Could you check a few things on this model? Use its own coordinates, in mm. Face numbers are marked on the shaded views. A direction names the side the tool comes from. Give positions to 0.01 mm unless a question says otherwise; leave off trailing zeros. Order: outer loops, then holes, each group sorted by start corner. A loop starts at its lowest first (then second) coordinate and runs counter-clockwise, first axis right, second up. Notation, with made-up numbers: (42, 66) -> (70, 66) arc R11 cw to (70, 76) -> close; hole circle Ø4 at (58.25, 11). An arc over 180 degrees is marked (long way). One line per item, written item: value.
```python
from build123d import *

# Parameters (mm, degrees)
EXTRUDE_1_DEPTH = 5
FILLET_1_R      = 0.5


with BuildPart() as part:
    # 草图1 → 凸台-拉伸1 (new body)
    with BuildSketch(Plane(origin=(0, 0, 0), x_dir=(1, 0, 0), z_dir=(0, 1, 0))):
        with BuildLine():
            ThreePointArc((-8.316516862, 5.552976435), (-7.071067812, 7.071067812), (-5.552976435, 8.316516862))
            Line((-5.552976435, 8.316516862), (-12.76036541, 15.523905838))
            Line((-12.76036541, 15.523905838), (-15.523905838, 12.76036541))
            Line((-15.523905838, 12.76036541), (-8.316516862, 5.552976435))
        make_face()
        with BuildLine():
            Line((-20, -1.954118176), (-9.807212762, -1.954118176))
            ThreePointArc((-9.807212762, -1.954118176), (-10, 0), (-9.807212762, 1.954118176))
            Line((-9.807212762, 1.954118176), (-20, 1.954118176))
            Line((-20, 1.954118176), (-20, -1.954118176))
        make_face()
        with BuildLine():
            Line((-12.76036541, -15.523905838), (-5.552976435, -8.316516862))
            ThreePointArc((-5.552976435, -8.316516862), (-7.071067812, -7.071067812), (-8.316516862, -5.552976435))
            Line((-8.316516862, -5.552976435), (-15.523905838, -12.76036541))
            Line((-15.523905838, -12.76036541), (-12.76036541, -15.523905838))
        make_face()
        with BuildLine():
            ThreePointArc((-1.954118176, -9.807212762), (-0.981802522, -9.951686481), (0, -10))
            Line((0, -10), (0, -2.5))
            ThreePointArc((0, -2.5), (-2.5, 0), (0, 2.5))
            Line((0, 2.5), (0, 10))
            ThreePointArc((0, 10), (-0.981802522, 9.951686481), (-1.954118176, 9.807212762))
            ThreePointArc((-1.954118176, 9.807212762), (-3.826834324, 9.238795325), (-5.552976435, 8.316516862))
            ThreePointArc((-5.552976435, 8.316516862), (-7.071067812, 7.071067812), (-8.316516862, 5.552976435))
            ThreePointArc((-8.316516862, 5.552976435), (-9.238795325, 3.826834324), (-9.807212762, 1.954118176))
            ThreePointArc((-9.807212762, 1.954118176), (-10, 0), (-9.807212762, -1.954118176))
            ThreePointArc((-9.807212762, -1.954118176), (-9.238795325, -3.826834324), (-8.316516862, -5.552976435))
            ThreePointArc((-8.316516862, -5.552976435), (-7.071067812, -7.071067812), (-5.552976435, -8.316516862))
            ThreePointArc((-5.552976435, -8.316516862), (-3.826834324, -9.238795325), (-1.954118176, -9.807212762))
        make_face()
        with BuildLine():
            Line((0, -2.5), (0, -10))
            ThreePointArc((0, -10), (0.981802522, -9.951686481), (1.954118176, -9.807212762))
            ThreePointArc((1.954118176, -9.807212762), (3.826834324, -9.238795325), (5.552976435, -8.316516862))
            ThreePointArc((5.552976435, -8.316516862), (7.071067812, -7.071067812), (8.316516862, -5.552976435))
            ThreePointArc((8.316516862, -5.552976435), (9.238795325, -3.826834324), (9.807212762, -1.954118176))
            ThreePointArc((9.807212762, -1.954118176), (9.951686481, -0.981802522), (10, 0))
            ThreePointArc((10, 0), (9.951686481, 0.981802522), (9.807212762, 1.954118176))
            ThreePointArc((9.807212762, 1.954118176), (9.238795325, 3.826834324), (8.316516862, 5.552976435))
            ThreePointArc((8.316516862, 5.552976435), (7.071067812, 7.071067812), (5.552976435, 8.316516862))
            ThreePointArc((5.552976435, 8.316516862), (3.826834324, 9.238795325), (1.954118176, 9.807212762))
            ThreePointArc((1.954118176, 9.807212762), (0.981802522, 9.951686481), (0, 10))
            Line((0, 10), (0, 2.5))
            ThreePointArc((0, 2.5), (1.767766953, 1.767766953), (2.5, 0))
            ThreePointArc((2.5, 0), (1.767766953, -1.767766953), (0, -2.5))
        make_face()
        with BuildLine():
            Line((0, 20), (0, 10))
            ThreePointArc((0, 10), (0.981802522, 9.951686481), (1.954118176, 9.807212762))
            Line((1.954118176, 9.807212762), (1.954118176, 20))
            Line((1.954118176, 20), (0, 20))
        make_face()
        with BuildLine():
            ThreePointArc((-1.954118176, 9.807212762), (-0.981802522, 9.951686481), (0, 10))
            Line((0, 10), (0, 20))
            Line((0, 20), (-1.954118176, 20))
            Line((-1.954118176, 20), (-1.954118176, 9.807212762))
        make_face()
        with BuildLine():
            Line((12.76036541, 15.523905838), (5.552976435, 8.316516862))
            ThreePointArc((5.552976435, 8.316516862), (7.071067812, 7.071067812), (8.316516862, 5.552976435))
            Line((8.316516862, 5.552976435), (15.523905838, 12.76036541))
            Line((15.523905838, 12.76036541), (12.76036541, 15.523905838))
        make_face()
        with BuildLine():
            ThreePointArc((10, 0), (9.951686481, -0.981802522), (9.807212762, -1.954118176))
            Line((9.807212762, -1.954118176), (20, -1.954118176))
            Line((20, -1.954118176), (20, 1.954118176))
            Line((20, 1.954118176), (9.807212762, 1.954118176))
            ThreePointArc((9.807212762, 1.954118176), (9.951686481, 0.981802522), (10, 0))
        make_face()
        with BuildLine():
            ThreePointArc((8.316516862, -5.552976435), (7.071067812, -7.071067812), (5.552976435, -8.316516862))
            Line((5.552976435, -8.316516862), (12.76036541, -15.523905838))
            Line((12.76036541, -15.523905838), (15.523905838, -12.76036541))
            Line((15.523905838, -12.76036541), (8.316516862, -5.552976435))
        make_face()
        with BuildLine():
            Line((-1.954118176, -20), (0, -20))
            Line((0, -20), (0, -10))
            ThreePointArc((0, -10), (-0.981802522, -9.951686481), (-1.954118176, -9.807212762))
            Line((-1.954118176, -9.807212762), (-1.954118176, -20))
        make_face()
        with BuildLine():
            Line((0, -10), (0, -20))
            Line((0, -20), (1.954118176, -20))
            Line((1.954118176, -20), (1.954118176, -9.807212762))
            ThreePointArc((1.954118176, -9.807212762), (0.981802522, -9.951686481), (0, -10))
        make_face()
    extrude(amount=EXTRUDE_1_DEPTH)

    # 圆角1
    fillet_1_edges = [part.edges().sort_by_distance(p)[0] for p in [
        (9.156670922, 5, 11.92021135),
        (14.142135624, 5, 14.142135624),
        (0, 5, -20),
        (11.92021135, 5, 9.156670922),
        (9.238795325, 5, 3.826834324),
        (14.903606381, 5, 1.954118176),
        (20, 5, 0),
        (14.903606381, 5, -1.954118176),
        (9.238795325, 5, -3.826834324),
        (11.92021135, 5, -9.156670922),
        (14.142135624, 5, -14.142135624),
        (9.156670922, 5, -11.92021135),
        (3.826834324, 5, -9.238795325),
        (-1.954118176, 5, -14.903606381),
        (-3.826834324, 5, -9.238795325),
        (-9.156670922, 5, -11.92021135),
        (-14.142135624, 5, -14.142135624),
        (-11.92021135, 5, -9.156670922),
        (-9.238795325, 5, -3.826834324),
        (-14.903606381, 5, -1.954118176),
        (-20, 5, 0),
        (-14.903606381, 5, 1.954118176),
        (1.954118176, 5, -14.903606381),
        (-9.238795325, 5, 3.826834324),
        (-11.92021135, 5, 9.156670922),
        (-14.142135624, 5, 14.142135624),
        (-9.156670922, 5, 11.92021135),
        (-3.826834324, 5, 9.238795325),
        (-1.954118176, 5, 14.903606381),
        (0, 5, 20),
        (1.954118176, 5, 14.903606381),
        (3.826834324, 5, 9.238795325),
    ]]
    fillet(fillet_1_edges, radius=FILLET_1_R)


solid = part.part
```
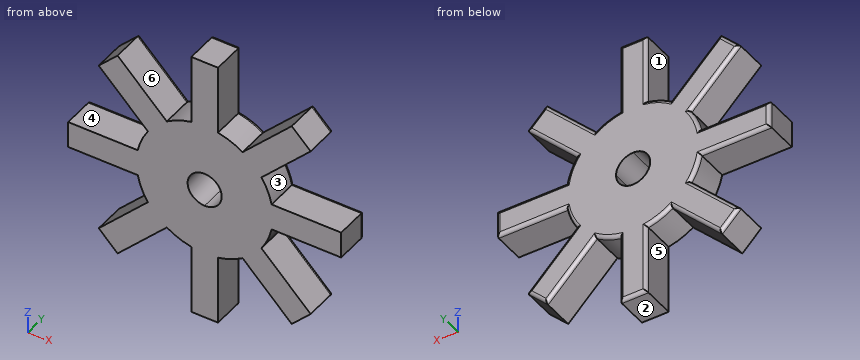
1) If I drill on line 1 along X through (y, z) = (3.9, -12); line 2 along X through (y, z) = (0.3, 13.5); line 3 along Z through (x, y) = (-15, 1.35), over which ranges is the centre line in solid material (lowest first)?
Answer below:
line 1: x = -14.76 to -9.24, -1.95 to 1.95, 9.24 to 14.76
line 2: x = -14.78 to -10.74, -1.95 to 1.95, 10.74 to 14.78
line 3: z = -13.28 to -12.24, -1.95 to 1.95, 12.24 to 13.28
2) We'd pull the mould along Z, two halves only. Please class the marked faces 1, 2 and 3: +Z half, -Z half, draft (parallel to the pull), parting line (faces both ways), or undercut.
Answer below:
face 1: draft
face 2: -Z half
face 3: undercut
3) Suppose I cut it at B-B, the plane x = -14. State how many separate pieces and enclosed holes the cut face has, then the cut area to 3 significant figures.
Answer below:
separate pieces: 3
enclosed holes: 0
area: 49.6 mm2
4) Suppose I cut it at A-A, the plane x = 16. Write out the boundary of the cut face in (y, z).
Answer below:
outline: (0, -1.95) -> (4.5, -1.95) arc R0.5 ccw to (5, -1.45) -> (5, 1.45) arc R0.5 ccw to (4.5, 1.95) -> (0, 1.95) -> close
5) For P1, Ø1.3, axis at x = -14.5, y = 2.5, coming from the -Z side; P2, Ø1, axis at y = 1, z = -4.5, coming from the +X side; P3, Ø1.3, axis at y = 2.5, z = -16, coming from the -X side, each with a flat end and sliding along its axis, tell me the tip position at first contact or that it passes through.
Answer below:
P1: stops at z = -14.43
P2: stops at x = 9.17
P3: stops at x = -12.93
6) For the marked faces 4, 5 and 6, which set-ups out of +Z, -Z, +X, -X, +Y, -Y let a thin tool reach every point of the face, with its end or its side?
Answer below:
face 4: -X, +Y, -Y
face 5: -Z, +Y, -Y
face 6: +Z, +Y, -Y
